Can you work these out from the drawing? Everything is in mm from the part's minimum corner. A direction names the side the tool comes from. Round coordinates to 2 decimals unless told otherwise and drop trailing zeros. Order: outer loops, then holes, each group sorted by start corner. A loop starts at its lowest first (then second) coordinate and runs counter-clockwise, first axis right, second up. Notation, with made-up numbers: (70, 78) - (101, 78) arc R9 cw to (101, 85) - close; hole circle Ø4 at (-3.75, 54). An arc over 180 degrees is marked (long way). Answer as a JSON object with one key per item and string values.
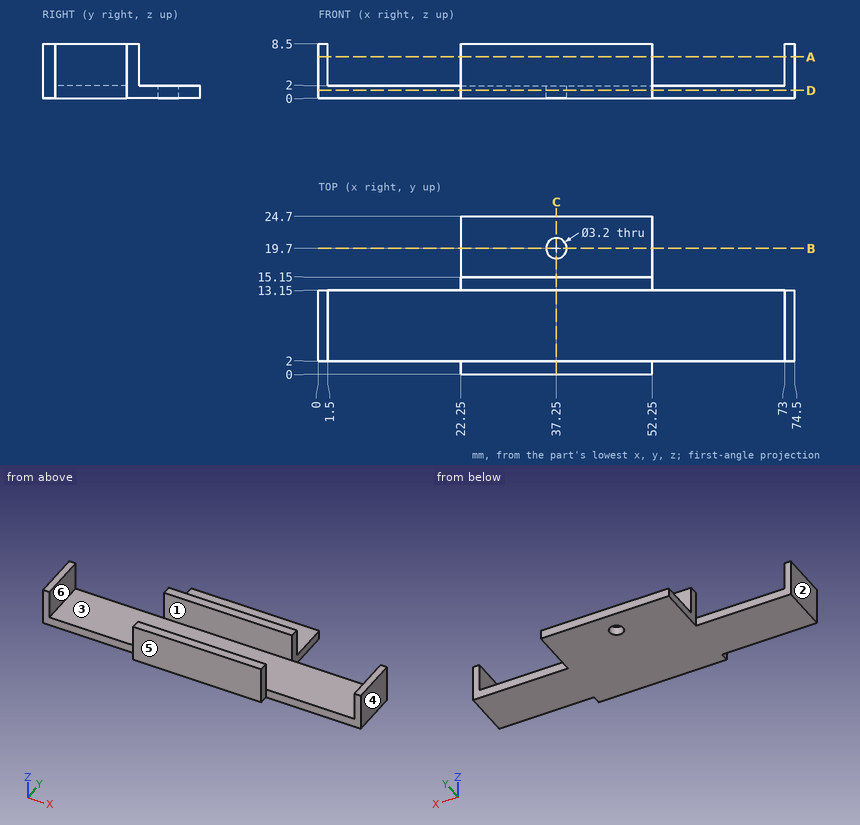
1. Imagine slicing it at D-D (z = 1.25). List the corners of the cut face in (x, y) for me.
Responses:
{"outline": "(0, 2) - (22.25, 2) - (22.25, 0) - (52.25, 0) - (52.25, 2) - (74.5, 2) - (74.5, 13.15) - (52.25, 13.15) - (52.25, 24.7) - (22.25, 24.7) - (22.25, 13.15) - (0, 13.15) - close; hole circle Ø3.2 at (37.25, 19.7)"}
2. Imagine slicing it at C-C (x = 37.25). List the corners of the cut face in (y, z) for me, plus the area to 3 significant figures.
Responses:
{"outline": "(0, 0) - (18.1, 0) - (18.1, 2) - (15.15, 2) - (15.15, 8.5) - (13.15, 8.5) - (13.15, 2) - (2, 2) - (2, 8.5) - (0, 8.5) - close; (21.3, 0) - (24.7, 0) - (24.7, 2) - (21.3, 2) - close", "area": "69.0 mm2"}
3. Imagine slicing it at B-B (y = 19.7). List the corners of the cut face in (x, z) for me, plus the area to 3 significant figures.
Responses:
{"outline": "(22.25, 0) - (35.65, 0) - (35.65, 2) - (22.25, 2) - close; (38.85, 0) - (52.25, 0) - (52.25, 2) - (38.85, 2) - close", "area": "53.6 mm2"}
4. If I drill on L1, parallel to Y at x = 34.5, z = 3; L2, parallel to X at y = 19.7, z = 0.6; L3, parallel to X at y = 7.75, z = 7, over which ranges is the centre line in solid material (lowest first)? Write a range as [from, to].
Responses:
{"L1": "[0, 2], [13.15, 15.15]", "L2": "[22.25, 35.65], [38.85, 52.25]", "L3": "[0, 1.5], [73, 74.5]"}
5. Imagine slicing it at A-A (z = 6.5). List the corners of the cut face in (x, y) for me, plus the area to 3 significant figures.
Responses:
{"outline": "(0, 2) - (1.5, 2) - (1.5, 13.15) - (0, 13.15) - close; (22.25, 0) - (52.25, 0) - (52.25, 2) - (22.25, 2) - close; (22.25, 13.15) - (52.25, 13.15) - (52.25, 15.15) - (22.25, 15.15) - close; (73, 2) - (74.5, 2) - (74.5, 13.15) - (73, 13.15) - close", "area": "153 mm2"}
6. For P1, Ø3, axis at x = 25, y = 18, coming from the -Z side; P2, Ø2.5, axis at x = 64.5, z = 2.5, coming from the -Y side; P3, Ø5, axis at y = 16, z = 1.5, coming from the -X side; P4, Ø5.5, axis at x = 23.5, y = 9.5, coming from the +Z side, each with a flat end and sliding along its axis, tell me the tip position at first contact or that it passes through.
Responses:
{"P1": "z = 0", "P2": "y = 2", "P3": "x = 22.25", "P4": "z = 2"}
7. For the marked faces 1 and 2, which set-ups out of +Z, -Z, +X, -X, +Y, -Y let a thin tool reach every point of the face, with its end or its side?
Responses:
{"face 1": "+Z", "face 2": "+Z, -Z, -X, +Y, -Y"}
8. Thinking about a two-plate mould opening in X: for the marked faces 3, 4, 5 and 6, which applies, pulls with the +X half, pulls with the -X half, needs draft (parallel to the pull), parting line crosses it, or undercut?
Responses:
{"face 3": "undercut", "face 4": "pulls with the +X half", "face 5": "needs draft", "face 6": "undercut"}
